The listing builds one solid part. Answer for the finished solid, in the listing's coordinates (mm). A direction names the side the tool comes from. Round coordinates to 2 decimals unless told otherwise and drop trailing zeros. Order: outer loops, then holes, each group sorted by start corner. A loop starts at its lowest first (then second) coordinate and runs counter-clockwise, first axis right, second up. Notation, with made-up numbers: M 81,69.5 L 124,69.5 A30 cw 124,103.5 Z; hole C 87,53 d4. An arc over 180 degrees is marked long. Write item = value, one per line. Start each with the question number.
(1) A cutting plane is placed at A-A, the plane z = 23. Determine the outline of the cut face in (x, y), and give its area (3 significant figures).
(2) Each of these flat-tipped pins is pushed along its axis until it touches: pin 1 (1 mm diameter, centred on x = 32, z = 15, fed in from -Y); pin 2 (5.5 mm diameter, centred on y = -11.5, z = 25, fed in from +X); pin 3 (4 mm diameter, centred on y = -9, z = 25.5, fed in from -X). Where does it stop, or does it pass through?
(3) For a pull along Z with two mould halves and no side action, classify faces 4 (the face through (25, -8, -1)), 5 (the face through (48, -8, 1)), 6 (the face through (25, -8, 0)), 7 (the face through (25.32, -15.4, 0.57)) as released by +Z, released by -Z, zero draft, split by the parting line, or undercut.
(4) Which of the six approach directions +Z, -Z, +X, -X, +Y, -Y give full straight-line access (tool end or side, diameter ignored) to faces 1 (the face through (24.83, -0.6, 25.43)), 2 (the face through (18, -12.8, 26.2)), 3 (the face through (24.9, -16.5, 22))?
(5) Straight lines are drawn through the part: probe 1 along Z at (x, y) = (22.5, -12); probe 2 along X at (y, z) = (-10, 1.25); probe 3 along Y at (x, z) = (47, 20.5). For each, find the intervals that lie inside material, in ascending order. Write a range as from..to.
(6) A cutting plane is placed at D-D, the plane z = 11.25. Determine the outline of the cut face in (x, y), and give its area (3 significant figures).
(7) A cutting plane is placed at B-B, the plane y = -12. Determine the outline of the cut face in (x, z), and give its area (3 significant figures).
from build123d import *

# Parameters (mm, degrees)
F1_DEPTH = 50
F2_W     = 2
F2_H     = 16
F3_DEPTH = 2
F4_W     = 18
F4_H     = 17
F5_DEPTH = 25
F7_R     = 5
F8_R     = 1.9999


# Not quite as in the source:
# - a fillet or chamfer is up to 0.001 mm smaller than in the source, because OpenCascade refuses the exact size
# - a feature of the source that left no trace in its solid (it failed there, or was rolled back) is left out


with BuildPart() as f1:
    # F0 (on Right) → F1 (new body)
    with BuildSketch(Plane.YZ):
        Polygon((0, 26), (0, 0), (-16, 0), (-16, 2), (-17, 2), (-17, -1), (1, -1), (1, 26), align=None)
        Polygon((-16, 26), (0, 26), (1, 26), (1, 27), (-17, 27), (-17, 22), (-16, 22), align=None)
    extrude(amount=F1_DEPTH)

    # F2 (on face) → F3 (join)
    with BuildSketch(Plane.XY):
        with Locations((1, -8)):
            Rectangle(F2_W, F2_H)
        with Locations((49, -8)):
            Rectangle(F2_W, F2_H)
    extrude(amount=F3_DEPTH)

    # F4 (on face) → F5 (cut)
    with BuildSketch(Plane.XY.offset(27)):
        with Locations((9, -8.5)):
            Rectangle(F4_W, F4_H)
        with Locations((41, -8.5)):
            Rectangle(F4_W, F4_H)
    extrude(amount=-F5_DEPTH, mode=Mode.SUBTRACT)

    # F7
    f7_edges = [f1.edges().sort_by_distance(p)[0] for p in [
        (32, 0, 26.5),
        (18, 0, 26.5),
    ]]
    fillet(f7_edges, radius=F7_R)

    # F8 (radius 2 in the source; OpenCascade refuses exactly that, so slightly less here)
    f8_edges = [f1.edges().sort_by_distance(p)[0] for p in [
        (25, -16, 0),
        (1, 0, 2),
        (25, 0, 26),
        (25, 0, 0),
        (49, 0, 2),
        (25, -16, 26),
    ]]
    fillet(f8_edges, radius=F8_R)


solid = f1.part
Reported:
q1.outline = M 0,0 L 50,0 L 50,1 L 0,1 Z; M 18,-17 L 32,-17 L 32,-16 L 18,-16 Z
q1.area = 64.0 mm²
q2.pin_1 = 0
q2.pin_2 = 32
q2.pin_3 = 18
q3.face_4 = released by -Z
q3.face_5 = zero draft
q3.face_6 = undercut
q3.face_7 = undercut
q4.face_1 = +X, -X
q4.face_2 = +Z, -X, -Y
q4.face_3 = +X, -X, -Y
q5.probe_1 = -1..0, 26..27
q5.probe_2 = 0..2, 48..50
q5.probe_3 = 0..1
q6.outline = M 0,0 L 50,0 L 50,1 L 0,1 Z
q6.area = 50.0 mm²
q7.outline = M 0,-1 L 50,-1 L 50,2 L 48,2 L 48,0 L 2,0 L 2,2 L 0,2 Z; M 18,26 L 32,26 L 32,27 L 18,27 Z
q7.area = 72.0 mm²
